from build123d import *

# Parameters (mm, degrees)
SKETCH1_W           = 211
SKETCH1_H           = 45
BOSS_EXTRUDE1_DEPTH = 4
CUT_EXTRUDE1_REACH  = 109.947
SKETCH2_W           = 95
SKETCH2_H           = 10
CUT_EXTRUDE2_REACH  = 109.947
SKETCH3_R           = 4.5
SKETCH3_W           = 20
SKETCH3_H           = 22.5
CUT_EXTRUDE3_DEPTH  = 4
CUT_EXTRUDE4_DEPTH  = 4
SKETCH7_R           = 5.771912947
CUT_EXTRUDE6_DEPTH  = 108.94674613
CUT_EXTRUDE7_REACH  = 109.947


with BuildPart() as part:
    # Sketch1 → Boss-Extrude1 (new body)
    with BuildSketch(Plane.XY):
        Rectangle(SKETCH1_W, SKETCH1_H)
    extrude(amount=BOSS_EXTRUDE1_DEPTH)

    # Sketch2 → Cut-Extrude1 (cut, up to next)
    with BuildSketch(Plane.XY.offset(4), mode=Mode.PRIVATE) as cut_extrude1_sk1:
        with Locations((-58, 17.5)):
            Rectangle(SKETCH2_W, SKETCH2_H)
    cut_extrude1_tool1 = extrude(cut_extrude1_sk1.sketch, amount=-CUT_EXTRUDE1_REACH, mode=Mode.PRIVATE) & part.part
    add(cut_extrude1_tool1.solids().sort_by_distance((-58, 17.5, 4))[0], mode=Mode.SUBTRACT)

    # Sketch3 → Cut-Extrude2 (cut, up to next)
    with BuildSketch(Plane.XY.offset(4), mode=Mode.PRIVATE) as cut_extrude2_sk1:
        with Locations((-44.5, -10.5)):
            Circle(SKETCH3_R)
    cut_extrude2_tool1 = extrude(cut_extrude2_sk1.sketch, amount=-CUT_EXTRUDE2_REACH, mode=Mode.PRIVATE) & part.part
    # Sketch3 → Cut-Extrude2 (cut, up to next)
    with BuildSketch(Plane.XY.offset(4), mode=Mode.PRIVATE) as cut_extrude2_sk2:
        with Locations((45.5, -11.25)):
            Rectangle(SKETCH3_W, SKETCH3_H)
        with Locations((45.5, -10.5)):
            Circle(SKETCH3_R, mode=Mode.SUBTRACT)
    cut_extrude2_tool2 = extrude(cut_extrude2_sk2.sketch, amount=-CUT_EXTRUDE2_REACH, mode=Mode.PRIVATE) & part.part
    add(cut_extrude2_tool1.solids().sort_by_distance((-44.5, -10.5, 4))[0], mode=Mode.SUBTRACT)
    add(cut_extrude2_tool2.solids().sort_by_distance((55.19896, -11.25, 4))[0], mode=Mode.SUBTRACT)


with BuildPart() as cut_extrude2_piece_1:
    # of the separate pieces the step leaves, piece 1, a body of its own (cut_extrude2_pieces)
    add(part.part.solids().sort_by_distance((-105.5, -22.5, 0))[0])

    # Sketch4 → Cut-Extrude3 (cut)
    with BuildSketch(Plane(origin=(0, 0, 0), x_dir=(-1, 0, 0), z_dir=(0, 0, -1))):
        Polygon((44.5, -22.5), (34.5, -22.5), (34.5, -2.5), (54.5, -2.5), (54.5, -22.5), align=None)
    extrude(amount=-CUT_EXTRUDE3_DEPTH, mode=Mode.SUBTRACT)

    # Sketch5 → Cut-Extrude4 (cut)
    with BuildSketch(Plane(origin=(0, 0, 0), x_dir=(-1, 0, 0), z_dir=(0, 0, -1))):
        with BuildLine():
            Line((101.601478709, -4.75), (88.754183798, -4.75))
            ThreePointArc((88.754183798, -4.75), (87.004183798, -6.5), (88.754183798, -8.25))
            Line((88.754183798, -8.25), (101.601478709, -8.25))
            ThreePointArc((101.601478709, -8.25), (103.351478709, -6.5), (101.601478709, -4.75))
        make_face()
    extrude(amount=-CUT_EXTRUDE4_DEPTH, mode=Mode.SUBTRACT)

    # Sketch8 → Cut-Extrude7 (cut, up to next)
    with BuildSketch(Plane(origin=(0, 0, 0), x_dir=(-1, 0, 0), z_dir=(0, 0, -1)), mode=Mode.PRIVATE) as cut_extrude7_sk1:
        with BuildLine():
            Line((-13.125491326, -8.25), (9.100552063, -8.25))
            ThreePointArc((9.100552063, -8.25), (10.850552063, -6.5), (9.100552063, -4.75))
            Line((9.100552063, -4.75), (-3.792824267, -4.75))
            Line((-3.792824267, -4.75), (-13.125491326, -4.75))
            ThreePointArc((-13.125491326, -4.75), (-14.875491326, -6.5), (-13.125491326, -8.25))
        make_face()
    cut_extrude7_tool1 = extrude(cut_extrude7_sk1.sketch, amount=-CUT_EXTRUDE7_REACH, mode=Mode.PRIVATE) & cut_extrude2_piece_1.part
    add(cut_extrude7_tool1.solids().sort_by_distance((2.01247, -6.5, 0))[0], mode=Mode.SUBTRACT)


with BuildPart() as cut_extrude2_piece_2:
    # of the separate pieces the step leaves, piece 2, a body of its own (cut_extrude2_pieces)
    add(part.part.solids().sort_by_distance((50, -10.5, 0))[0])

    # Sketch7 → Cut-Extrude6 (cut, through all)
    with BuildSketch(Plane(origin=(0, 0, 0), x_dir=(-1, 0, 0), z_dir=(0, 0, -1))):
        with Locations((-45.5, -10.5)):
            Circle(SKETCH7_R)
    extrude(amount=-CUT_EXTRUDE6_DEPTH, mode=Mode.SUBTRACT)


solid = cut_extrude2_piece_1.part
Could you check a few things on this model? Use its own coordinates, in mm. A direction names the side the tool comes from. Coordinates: 2 decimals unless noted, no trailing zeros. Order: outer loops, then holes, each group sorted by start corner. A loop starts at its lowest first (then second) coordinate and runs counter-clockwise, first axis right, second up. Notation, with made-up numbers: (23, 44.25) - (42, 44.25) arc R26 cw to (42, 59.25) - close; hole circle Ø3 at (60.25, 21.25). An arc over 180 degrees is marked (long way). Answer in a Markdown table with one row per item. Add a question column.
(1) On a 3-axis mill with a long thin cutter (end or side, diameter ignored), from which of +Z, -Z, +X, -X, +Y, -Y can I reach the whole of each face in a straight line? I mean faces 5 (the face through (-44, -2.5, 2)), 6 (the face through (-59, 12.5, 2)), 7 (the face through (-95, -8.25, 2)). Say none if no direction works.
(2) If we section it at A-A, the plane y = -6.5: Please give me the cut outline in (x, z), then the cut area to 3 significant figures.
(3) If we section it at D-D, the plane y = -18.5: Please give me the cut outline in (x, z), then the cut area to 3 significant figures.
(4) If we section it at B-B, the plane z = 2.7: Please give me the cut outline in (x, y), then the cut area to 3 significant figures.
(5) I need wall thicknesses on L1, parallel to X at y = -11.5, z = 3.4; L2, parallel to X at y = -5, z = 3; L3, parallel to Y at x = -59, z = 1.05. Which ranges of each line are inside material? Lowest first, please.
(6) If we mould it in two halves opening along X, with no side actions, what happens to faces 1 (the face through (-105.5, -5, 2)), 2 (the face through (-1, 0, 4)), 3 (the face through (35.5, -11, 2)), 4 (the face through (14.875, -6.462, 1.972))? For each: released by +X, released by -X, zero draft, split by the parting line, or undercut.
(7) If we section it at C-C, the plane x = -6: Please give me the cut outline in (y, z).
(8) Will these pins go through, and if not, where does the flat tip stop? pin 1 (1.2 mm diameter, centred on y = 19, z = 2, fed in from -X); pin 2 (2 mm diameter, centred on x = -94, z = 2.5, fed in from +Y); pin 3 (2 mm diameter, centred on x = 47.5, z = 3, fed in from -Y).
Results are:
| question | item | result |
|---|---|---|
| 1 | face 5 | +Z, -Z, -Y |
| 1 | face 6 | +Z, -Z, -X, +Y |
| 1 | face 7 | +Z, -Z |
| 2 | outline | (-105.5, 0) - (-103.35, 0) - (-103.35, 4) - (-105.5, 4) - close; (-87, 0) - (-54.5, 0) - (-54.5, 4) - (-87, 4) - close; (-34.5, 0) - (-10.85, 0) - (-10.85, 4) - (-34.5, 4) - close; (14.88, 0) - (35.5, 0) - (35.5, 4) - (14.88, 4) - close; (55.5, 0) - (105.5, 0) - (105.5, 4) - (55.5, 4) - close |
| 2 | area | 516 mm2 |
| 3 | outline | (-105.5, 0) - (-54.5, 0) - (-54.5, 4) - (-105.5, 4) - close; (-34.5, 0) - (35.5, 0) - (35.5, 4) - (-34.5, 4) - close; (55.5, 0) - (105.5, 0) - (105.5, 4) - (55.5, 4) - close |
| 3 | area | 684 mm2 |
| 4 | outline | (-105.5, -22.5) - (-54.5, -22.5) - (-54.5, -2.5) - (-34.5, -2.5) - (-34.5, -22.5) - (35.5, -22.5) - (35.5, 0) - (55.5, 0) - (55.5, -22.5) - (105.5, -22.5) - (105.5, 22.5) - (-10.5, 22.5) - (-10.5, 12.5) - (-105.5, 12.5) - close; hole (-101.6, -8.25) - (-88.75, -8.25) arc R1.75 ccw to (-88.75, -4.75) - (-101.6, -4.75) arc R1.75 ccw to start; hole (-9.1, -8.25) - (13.13, -8.25) arc R1.75 ccw to (13.13, -4.75) - (-9.1, -4.75) arc R1.75 ccw to start |
| 4 | area | 7,550 mm2 |
| 5 | L1 | x = -105.5 to -54.5, -34.5 to 35.5, 55.5 to 105.5 |
| 5 | L2 | x = -105.5 to -102.5, -87.85 to -54.5, -34.5 to -10, 14.03 to 35.5, 55.5 to 105.5 |
| 5 | L3 | y = -22.5 to 12.5 |
| 6 | face 1 | released by -X |
| 6 | face 2 | zero draft |
| 6 | face 3 | undercut |
| 6 | face 4 | undercut |
| 7 | outline | (-22.5, 0) - (-8.25, 0) - (-8.25, 4) - (-22.5, 4) - close; (-4.75, 0) - (22.5, 0) - (22.5, 4) - (-4.75, 4) - close |
| 8 | pin 1 | stops at x = -10.5 |
| 8 | pin 2 | stops at y = 12.5 |
| 8 | pin 3 | stops at y = 0 |
